from build123d import *

# Parameters (mm, degrees)
BASE_FLANGE1_DEPTH = 150
CUT_EXTRUDE1_DEPTH = 226


# Sheet-metal steps are written as plain solids
with BuildPart() as part:
    # Sketch1 → Base-Flange1 (new body)
    with BuildSketch(Plane.XY):
        with BuildLine():
            Line((72, -72), (72, 71.2634))
            ThreePointArc((72, 71.2634), (71.784254855, 71.784254855), (71.2634, 72))
            Line((71.2634, 72), (-71.2634, 72))
            ThreePointArc((-71.2634, 72), (-71.784254855, 71.784254855), (-72, 71.2634))
            Line((-72, 71.2634), (-72, -72))
            Line((-72, -72), (-75, -72))
            Line((-75, -72), (-75, 71.2634))
            ThreePointArc((-75, 71.2634), (-73.905575199, 73.905575199), (-71.2634, 75))
            Line((-71.2634, 75), (71.2634, 75))
            ThreePointArc((71.2634, 75), (73.905575199, 73.905575199), (75, 71.2634))
            Line((75, 71.2634), (75, -72))
            Line((75, -72), (72, -72))
        make_face()
    extrude(amount=BASE_FLANGE1_DEPTH)

    # Sketch6 → Cut-Extrude1 (cut, through all)
    with BuildSketch(Plane.ZY.offset(75)):
        Polygon((75, -72), (150, 31.405620606), (170.305781078, 31.405620606), (170.305781078, -96.262552323), (75, -96.262552323), align=None)
    extrude(amount=-CUT_EXTRUDE1_DEPTH, mode=Mode.SUBTRACT)


solid = part.part
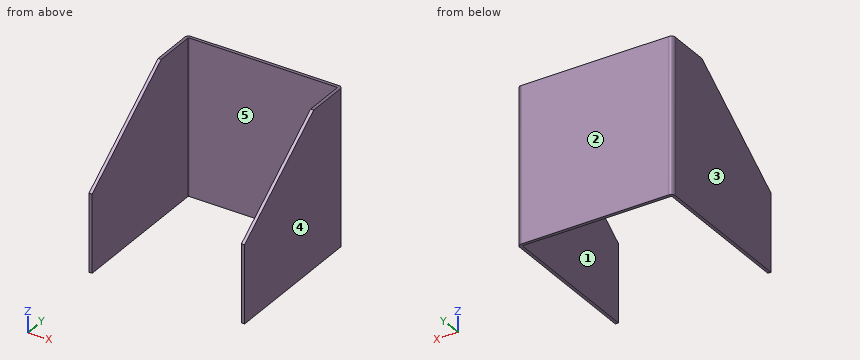
The listing builds one solid part. Answer for the finished solid, in the listing's coordinates (mm). Face numbers are marked on the shaded views. A direction names the side the tool comes from. Round coordinates to 2 decimals unless told otherwise and drop trailing zeros. Order: outer loops, then holes, each group sorted by start corner. A loop starts at its lowest first (then second) coordinate and runs counter-clockwise, first axis right, second up. Notation, with made-up numbers: (85.25, -12) -> (104.25, -12) arc R31 cw to (104.25, 22) -> close; hole circle Ø5 at (83, 33). An arc over 180 degrees is marked (long way). One line per item, written item: value.
Item 1: Find section D-D, the plane y = 0. Give the vertices of the cut face in (x, z), then the cut area to 3 significant figures.
Taken from the geometry:
outline: (-75, 0) -> (-72, 0) -> (-72, 127.22) -> (-75, 127.22) -> close; (72, 0) -> (75, 0) -> (75, 127.22) -> (72, 127.22) -> close
area: 763 mm2
Item 2: For a pull along X with two mould halves and no side action, classify the marked faces 1, 2 and 3 as released by +X, released by -X, zero draft, split by the parting line, or undercut.
Taken from the geometry:
face 1: undercut
face 2: zero draft
face 3: released by -X
Item 3: Find section C-C, the plane x = -11.5. Give the vertices of the cut face in (y, z).
Taken from the geometry:
outline: (72, 0) -> (75, 0) -> (75, 150) -> (72, 150) -> close
Item 4: Find section B-B, the plane z = 23. Give the vertices of the cut face in (x, y).
Taken from the geometry:
outline: (-75, -72) -> (-72, -72) -> (-72, 71.26) arc R0.74 cw to (-71.26, 72) -> (71.26, 72) arc R0.74 cw to (72, 71.26) -> (72, -72) -> (75, -72) -> (75, 71.26) arc R3.74 ccw to (71.26, 75) -> (-71.26, 75) arc R3.74 ccw to (-75, 71.26) -> close
Item 5: Find section A-A, the plane y = -39.5. Give the vertices of the cut face in (x, z).
Taken from the geometry:
outline: (-75, 0) -> (-72, 0) -> (-72, 98.57) -> (-75, 98.57) -> close; (72, 0) -> (75, 0) -> (75, 98.57) -> (72, 98.57) -> close
Item 6: For the marked faces 4 and 5, determine the directions among +Z, -Z, +X, -X, +Y, -Y from which every point of the face is accessible in a straight line to the end or side of a thin tool.
Taken from the geometry:
face 4: +Z, -Z, +X, +Y, -Y
face 5: +Z, -Z, -Y
Item 7: Given P1, Ø12, axis at x = 51.5, z = 79, coming from the -Y side; P2, Ø12, axis at y = -4, z = 125, coming from the +X side, each flat-ended and moving along its own axis, determine where each tip first touches the part or whether it passes through.
Taken from the geometry:
P1: stops at y = 72
P2: stops at x = 75
Item 8: Straight lines are drawn through the part: L1, parallel to X at y = -59, z = 7.5; L2, parallel to Y at x = 33.5, z = 21.5. For each, find the intervals that lie inside material, in ascending order.
Taken from the geometry:
L1: x = -75 to -72, 72 to 75
L2: y = 72 to 75
